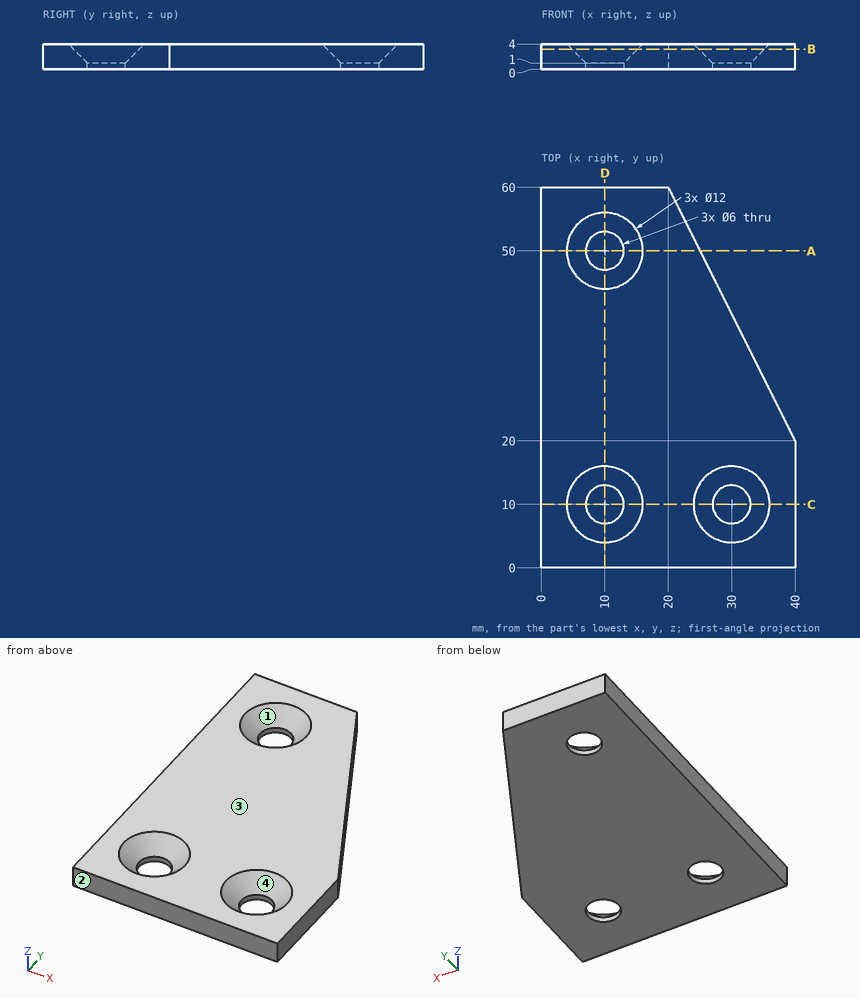
Could you check a few things on this drawing? It's one solid part, dimensions in mm from its lowest x, y, z. Round coordinates to 2 decimals unless told otherwise and drop trailing zeros. Loops run counter-clockwise (first coordinate to the right, second up) from the corner with the lowest first, then second, coordinate; pieces in that order, holes last. Notation, with made-up numbers: M 66,78 L 72,78 A20 ccw 72,104 Z; hole C -30,37 d7. An arc over 180 degrees is marked long. Write item = value, one per line. Start each with the question number.
(1) I need wall thicknesses on line 1 along Y through (x, z) = (10, 0.85); line 2 along X through (y, z) = (13.5, 3.8); line 3 along Y through (x, z) = (30, 0.6). Which ranges of each line are inside material? Lowest first, please.
(2) If we mould it in two halves opening along Y, with no side actions, what happens to the marked faces 1, 2, 3 and 4? For each: released by +Y, released by -Y, zero draft, split by the parting line, or undercut.
(3) Suppose I cut it at B-B on z = 3.2. Write out the boundary of the cut face in (x, y).
(4) Suppose I cut it at D-D on x = 10. Write out the boundary of the cut face in (y, z).
(5) Suppose I cut it at A-A on y = 50. Write out the boundary of the cut face in (x, z), plus the area to 3 significant figures.
(6) I'm going to push flat-ended pins straight in: P1, Ø9.5, axis at x = 10, y = 10, coming from the +Z side; P2, Ø2, axis at x = 34.5, z = 2, coming from the +Y side; P3, Ø1, axis at y = 47, z = 0.5, coming from the +X side. Where does each tip first touch, or does it pass through?
(7) Suppose I cut it at C-C on y = 10. Write out the boundary of the cut face in (x, z).
Answer block:
q1.line_1 = 0 to 7, 13 to 47, 53 to 60
q1.line_2 = 0 to 5.38, 14.62 to 25.38, 34.62 to 40
q1.line_3 = 0 to 7, 13 to 40
q2.face_1 = undercut
q2.face_2 = released by -Y
q2.face_3 = zero draft
q2.face_4 = undercut
q3.outline = M 0,0 L 40,0 L 40,20 L 20,60 L 0,60 Z; hole C 10,10 d10.4; hole C 10,50 d10.4; hole C 30,10 d10.4
q4.outline = M 0,0 L 7,0 L 7,1 L 4,4 L 0,4 Z; M 13,0 L 47,0 L 47,1 L 44,4 L 16,4 L 13,1 Z; M 53,0 L 60,0 L 60,4 L 56,4 L 53,1 Z
q5.outline = M 0,0 L 7,0 L 7,1 L 4,4 L 0,4 Z; M 13,0 L 25,0 L 25,4 L 16,4 L 13,1 Z
q5.area = 67.0 mm²
q6.P1 = 2.75
q6.P2 = 33
q6.P3 = 26.75
q7.outline = M 0,0 L 7,0 L 7,1 L 4,4 L 0,4 Z; M 13,0 L 27,0 L 27,1 L 24,4 L 16,4 L 13,1 Z; M 33,0 L 40,0 L 40,4 L 36,4 L 33,1 Z
